Check sheet for the modelled part. Datum: model origin and axes. Units: mm. Round coordinates to 2 decimals unless told otherwise and drop trailing zeros. Order: outer loops, then holes, each group sorted by start corner. A loop starts at its lowest first (then second) coordinate and runs counter-clockwise, first axis right, second up.
(1) Sectioned sample at A-A, the plane z = 0. Enter the section's corners in (x, y).
(2) Mould release check, pull along X, two halves, no side actions. Record for faces 1 (the cylindrical face through (0.66, -0.07, -14.985)), 2 (the flat face through (-1, -3, 25)), 3 (the cylindrical face through (-10.648, 2.465, -13.887)), 4 (the flat face through (100, -3, 0)): released by +X, released by -X, zero draft, split by the parting line, or undercut.
(3) Sectioned sample at C-C, the plane y = 1.75. Enter the section's corners in (x, z).
(4) Sectioned sample at D-D, the plane z = 21. Enter the section's corners in (x, y).
(5) Thickness scan on probe 1 along X at (y, z) = (-2.5, 0); probe 2 along Y at (x, z) = (85, 2); probe 3 along X at (y, z) = (1.5, 0). Record the ranges inside material, lowest first.
(6) Sectioned sample at B-B, the plane x = 0. Enter the section's corners in (y, z), and give its area (3 significant figures).
(7) Depth check by flat-ended pin: pin 1 (1 mm diameter, centred on x = -16.5, z = 19, fed in from +Y); pin 2 (1.5 mm diameter, centred on x = -40.5, y = 0.5, fed in from -Z). Enter the tip coordinate at first touch or a pass-through.
```python
from build123d import *

# Parameters (mm, degrees)
SKETCH1_R           = 17.5
SKETCH1_R_2         = 15
BOSS_EXTRUDE1_DEPTH = 5
BOSS_EXTRUDE2_START = -5
SKETCH1_3_W         = 200
SKETCH1_3_H         = 50
SKETCH1_3_R         = 17.5
SKETCH1_3_R_2       = 15
BOSS_EXTRUDE2_DEPTH = 5


with BuildPart() as part:
    # Sketch1 → Boss-Extrude1 (new body)
    with BuildSketch(Plane(origin=(0, 0, 0), x_dir=(1, 0, 0), z_dir=(0, 1, 0))):
        with Locations(Location((0, 0, 0), (0, 0, 270))):
            Circle(SKETCH1_R)
        with Locations(Location((0, 0, 0), (0, 0, 270))):
            Circle(SKETCH1_R_2, mode=Mode.SUBTRACT)
    extrude(amount=BOSS_EXTRUDE1_DEPTH)

    # Sketch1_3 → Boss-Extrude2 (add)
    # profile 1 of 2: a face of its own
    with BuildSketch(Plane(origin=(0, 0, 0), x_dir=(1, 0, 0), z_dir=(0, 1, 0)).offset(BOSS_EXTRUDE2_START)):
        Rectangle(SKETCH1_3_W, SKETCH1_3_H)
        with Locations(Location((0, 0, 0), (0, 0, 270))):
            Circle(SKETCH1_3_R, mode=Mode.SUBTRACT)
    # profile 2 of 2: a face of its own
    with BuildSketch(Plane(origin=(0, 0, 0), x_dir=(1, 0, 0), z_dir=(0, 1, 0)).offset(BOSS_EXTRUDE2_START)):
        with Locations(Location((0, 0, 0), (0, 0, 270))):
            Circle(SKETCH1_3_R)
        with Locations(Location((0, 0, 0), (0, 0, 270))):
            Circle(SKETCH1_3_R_2, mode=Mode.SUBTRACT)
    extrude(amount=BOSS_EXTRUDE2_DEPTH)


solid = part.part
```
Derived:
1. outline: (-100, -5) - (-15, -5) - (-15, 5) - (-17.5, 5) - (-17.5, 0) - (-100, 0) - close; (15, -5) - (100, -5) - (100, 0) - (17.5, 0) - (17.5, 5) - (15, 5) - close
2. face 1: undercut
2. face 2: zero draft
2. face 3: split by the parting line
2. face 4: released by +X
3. outline: circle Ø35 at (0, 0); hole circle Ø30 at (0, 0)
4. outline: (-100, -5) - (100, -5) - (100, 0) - (-100, 0) - close
5. probe 1: x = -100 to -15, 15 to 100
5. probe 2: y = -5 to 0
5. probe 3: x = -17.5 to -15, 15 to 17.5
6. outline: (-5, -25) - (0, -25) - (0, -17.5) - (5, -17.5) - (5, -15) - (-5, -15) - close; (-5, 15) - (5, 15) - (5, 17.5) - (0, 17.5) - (0, 25) - (-5, 25) - close
6. area: 125 mm2
7. pin 1: stops at y = 0
7. pin 2: stops at z = -25
